Input: part model. Units: mm. Frame: model coordinates. Give positions to 0.01 mm unless a question says otherwise; leave off trailing zeros. Write each loop counter-clockwise with the first axis right and the second up, starting at its lowest first coordinate (ties: lowest second). Pieces come first, ordered by that corner, then holes.
```python
from build123d import *

# Parameters (mm, degrees)
F0_W     = 112.25
F0_H     = 107.75
F0_R     = 2.25
F0_R_2   = 3.275
F0_W_2   = 10
F0_H_2   = 2
F0_R_3   = 3
F0_R_4   = 8.45
F0_W_3   = 80.22
F0_H_3   = 53.05
F1_DEPTH = 2
F2_W     = 6
F2_H     = 9.375001
F2_H_2   = 10
F2_W_2   = 10
F2_H_3   = 6
F3_DEPTH = 3


with BuildPart() as f1:
    # F0 (on Top) → F1 (new body)
    with BuildSketch(Plane.XY):
        with Locations((56.125, 53.875)):
            Rectangle(F0_W, F0_H)
        with Locations((3.5, 3.5)):
            Circle(F0_R, mode=Mode.SUBTRACT)
        with Locations((17.59, 21.63)):
            Circle(F0_R_2, mode=Mode.SUBTRACT)
        with Locations((74, 9.726001)):
            Rectangle(F0_W_2, F0_H_2, mode=Mode.SUBTRACT)
        with Locations((60, 18.3)):
            Circle(F0_R_3, mode=Mode.SUBTRACT)
        with Locations((73.933571, 13.617334)):
            Rectangle(F0_W_2, F0_H_2, mode=Mode.SUBTRACT)
        with Locations((73.867143, 17.508667)):
            Rectangle(F0_W_2, F0_H_2, mode=Mode.SUBTRACT)
        with Locations((73.800714, 21.4)):
            Rectangle(F0_W_2, F0_H_2, mode=Mode.SUBTRACT)
        with Locations((73.734285, 25.291333)):
            Rectangle(F0_W_2, F0_H_2, mode=Mode.SUBTRACT)
        with Locations((108.75, 3.5)):
            Circle(F0_R, mode=Mode.SUBTRACT)
        with Locations((92.23, 18.3)):
            Circle(F0_R_4, mode=Mode.SUBTRACT)
        with Locations((55.86, 62.525)):
            Rectangle(F0_W_3, F0_H_3, mode=Mode.SUBTRACT)
        with Locations((3.5, 104.25)):
            Circle(F0_R, mode=Mode.SUBTRACT)
        with Locations((108.75, 104.25)):
            Circle(F0_R, mode=Mode.SUBTRACT)
    extrude(amount=F1_DEPTH)

    # F2 (on face) → F3 (join)
    with BuildSketch(Plane.XY.offset(2)):
        with Locations((112.25, 53.5575)):
            Rectangle(F2_W, F2_H)
        with Locations((0, 53.87)):
            Rectangle(F2_W, F2_H_2)
        with Locations((56.13, 107.75)):
            Rectangle(F2_W_2, F2_H_3)
        with Locations((56.13, 0)):
            Rectangle(F2_W_2, F2_H_3)
    extrude(amount=F3_DEPTH)


solid = f1.part
```
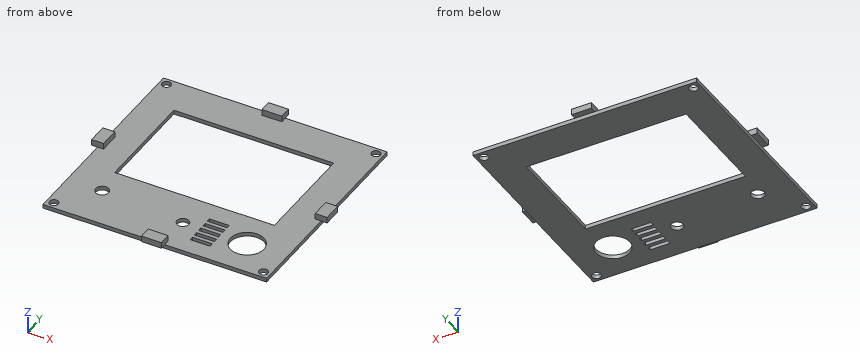
Item 1: Section D-D (z = 3.55). Return loops of the section in (x, y) (3 decimals).
Item 2: Section A-A (x = 74). Return loops of the section in (y, z), and give its area (3 significant figures).
Item 3: Pin query (flat end, axial travel): pin 1 (1 mm diameter, centred on y = 25, z = 1, fed in from +X); pin 2 (1.6 mm diameter, centred on x = 76, z = 1.5, fed in from -Y); pin 3 (8 mm diameter, centred on x = 83, y = 29.5, fed in from +Z); pin 4 (6 mm diameter, centred on x = 89, y = 40, fed in from -Z). Return the tip coordinate at first contact, or that it passes through.
Item 4: Ray query, line 1 (Y direction, x = 60, z = 0.65); line 2 (Y direction, x = 3.5, z = 0.65); line 3 (X direction, y = 73.5, z = 1). Return the intervals inside material, ascending.
Item 5: Section C-C (x = 17.59). Return loops of the section in (y, z) (3 decimals).
Item 6: Section B-B (y = 75.5). Return loops of the section in (x, z).
Solved:
1. outline: (-3, 48.87) - (3, 48.87) - (3, 58.87) - (-3, 58.87) - close; (51.13, -3) - (61.13, -3) - (61.13, 3) - (51.13, 3) - close; (51.13, 104.75) - (61.13, 104.75) - (61.13, 110.75) - (51.13, 110.75) - close; (109.25, 48.87) - (115.25, 48.87) - (115.25, 58.245) - (109.25, 58.245) - close
2. outline: (0, 0) - (8.73, 0) - (8.73, 2) - (0, 2) - close; (10.73, 0) - (12.62, 0) - (12.62, 2) - (10.73, 2) - close; (14.62, 0) - (16.51, 0) - (16.51, 2) - (14.62, 2) - close; (18.51, 0) - (20.4, 0) - (20.4, 2) - (18.51, 2) - close; (22.4, 0) - (24.29, 0) - (24.29, 2) - (22.4, 2) - close; (26.29, 0) - (36, 0) - (36, 2) - (26.29, 2) - close; (89.05, 0) - (107.75, 0) - (107.75, 2) - (89.05, 2) - close
2. area: 89.4 mm2
3. pin 1: stops at x = 112.25
3. pin 2: stops at y = 0
3. pin 3: stops at z = 2
3. pin 4: passes through
4. line 1: y = 0 to 15.3, 21.3 to 36, 89.05 to 107.75
4. line 2: y = 0 to 1.25, 5.75 to 102, 106.5 to 107.75
4. line 3: x = 0 to 15.75, 95.97 to 112.25
5. outline: (0, 0) - (18.355, 0) - (18.355, 2) - (0, 2) - close; (24.905, 0) - (36, 0) - (36, 2) - (24.905, 2) - close; (89.05, 0) - (107.75, 0) - (107.75, 2) - (89.05, 2) - close
6. outline: (0, 0) - (15.75, 0) - (15.75, 2) - (0, 2) - close; (95.97, 0) - (112.25, 0) - (112.25, 2) - (95.97, 2) - close
